```python
from build123d import *

# Parameters (mm, degrees)
BOSS_EXTRUDE3_DEPTH = 1
BOSS_EXTRUDE4_DEPTH = 3


with BuildPart() as part:
    # Sketch1 → Boss-Extrude3 (new body)
    with BuildSketch(Plane(origin=(0, 0, 0), x_dir=(1, 0, 0), z_dir=(0, 1, 0))):
        Polygon((362.222534427, 19.965180646), (284.852100337, -114.072137645), (439.598290008, -114.060221421), align=None)
        with BuildLine():
            Line((363.912669034, -12.581193275), (364.023092144, -12.093538954))
            ThreePointArc((364.023092144, -12.093538954), (365.725004108, -13.032245467), (366.663710621, -14.734157431))
            Line((366.663710621, -14.734157431), (366.1760563, -14.844580541))
            ThreePointArc((366.1760563, -14.844580541), (366.250130374, -15.507119201), (366.1760563, -16.169657861))
            Line((366.1760563, -16.169657861), (366.663710621, -16.280080971))
            ThreePointArc((366.663710621, -16.280080971), (365.725004108, -17.981992935), (364.023092144, -18.920699448))
            Line((364.023092144, -18.920699448), (363.912669034, -18.433045127))
            ThreePointArc((363.912669034, -18.433045127), (363.250130374, -18.507119201), (362.587591714, -18.433045127))
            Line((362.587591714, -18.433045127), (362.477168604, -18.920699448))
            ThreePointArc((362.477168604, -18.920699448), (360.77525664, -17.981992935), (359.836550127, -16.280080971))
            Line((359.836550127, -16.280080971), (360.324204448, -16.169657861))
            ThreePointArc((360.324204448, -16.169657861), (360.250130374, -15.507119201), (360.324204448, -14.844580541))
            Line((360.324204448, -14.844580541), (359.836550127, -14.734157431))
            ThreePointArc((359.836550127, -14.734157431), (360.77525664, -13.032245467), (362.477168604, -12.093538954))
            Line((362.477168604, -12.093538954), (362.587591714, -12.581193275))
            ThreePointArc((362.587591714, -12.581193275), (363.250130374, -12.507119201), (363.912669034, -12.581193275))
        make_face(mode=Mode.SUBTRACT)
        with BuildLine():
            ThreePointArc((313.830794955, -100.2988546), (312.128882991, -99.360148087), (311.190176478, -97.658236123))
            Line((311.190176478, -97.658236123), (311.677830799, -97.547813013))
            ThreePointArc((311.677830799, -97.547813013), (311.603756725, -96.885274353), (311.677830799, -96.222735693))
            Line((311.677830799, -96.222735693), (311.190176478, -96.112312583))
            ThreePointArc((311.190176478, -96.112312583), (312.128882991, -94.410400619), (313.830794955, -93.471694106))
            Line((313.830794955, -93.471694106), (313.941218065, -93.959348427))
            ThreePointArc((313.941218065, -93.959348427), (314.603756725, -93.885274353), (315.266295385, -93.959348427))
            Line((315.266295385, -93.959348427), (315.376718495, -93.471694106))
            ThreePointArc((315.376718495, -93.471694106), (317.078630459, -94.410400619), (318.017336972, -96.112312583))
            Line((318.017336972, -96.112312583), (317.529682651, -96.222735693))
            ThreePointArc((317.529682651, -96.222735693), (317.603756725, -96.885274353), (317.529682651, -97.547813013))
            Line((317.529682651, -97.547813013), (318.017336972, -97.658236123))
            ThreePointArc((318.017336972, -97.658236123), (317.078630459, -99.360148087), (315.376718495, -100.2988546))
            Line((315.376718495, -100.2988546), (315.266295385, -99.811200279))
            ThreePointArc((315.266295385, -99.811200279), (314.603756725, -99.885274353), (313.941218065, -99.811200279))
            Line((313.941218065, -99.811200279), (313.830794955, -100.2988546))
        make_face(mode=Mode.SUBTRACT)
        with BuildLine():
            ThreePointArc((406.858805843, -97.563455036), (407.797512356, -95.861543072), (409.49942432, -94.922836559))
            Line((409.49942432, -94.922836559), (409.60984743, -95.41049088))
            ThreePointArc((409.60984743, -95.41049088), (410.27238609, -95.336416806), (410.93492475, -95.41049088))
            Line((410.93492475, -95.41049088), (411.04534786, -94.922836559))
            ThreePointArc((411.04534786, -94.922836559), (412.747259824, -95.861543072), (413.685966337, -97.563455036))
            Line((413.685966337, -97.563455036), (413.198312016, -97.673878146))
            ThreePointArc((413.198312016, -97.673878146), (413.27238609, -98.336416806), (413.198312016, -98.998955466))
            Line((413.198312016, -98.998955466), (413.685966337, -99.109378576))
            ThreePointArc((413.685966337, -99.109378576), (412.747259824, -100.81129054), (411.04534786, -101.749997053))
            Line((411.04534786, -101.749997053), (410.93492475, -101.262342732))
            ThreePointArc((410.93492475, -101.262342732), (410.27238609, -101.336416806), (409.60984743, -101.262342732))
            Line((409.60984743, -101.262342732), (409.49942432, -101.749997053))
            ThreePointArc((409.49942432, -101.749997053), (407.797512356, -100.81129054), (406.858805843, -99.109378576))
            Line((406.858805843, -99.109378576), (407.346460164, -98.998955466))
            ThreePointArc((407.346460164, -98.998955466), (407.272389017, -98.332225876), (407.348322685, -97.665705839))
            Line((407.348322685, -97.665705839), (406.858805843, -97.563455036))
        make_face(mode=Mode.SUBTRACT)
    extrude(amount=BOSS_EXTRUDE3_DEPTH)

    # Sketch1<15> → Boss-Extrude4 (add)
    with BuildSketch(Plane(origin=(0, 0, 0), x_dir=(1, 0, 0), z_dir=(0, 1, 0))):
        with BuildLine():
            Line((315.266295385, -99.811200279), (315.376718495, -100.2988546))
            ThreePointArc((315.376718495, -100.2988546), (317.078630459, -99.360148087), (318.017336972, -97.658236123))
            Line((318.017336972, -97.658236123), (317.529682651, -97.547813013))
            ThreePointArc((317.529682651, -97.547813013), (316.725077068, -99.006594697), (315.266295385, -99.811200279))
        make_face()
        with BuildLine():
            ThreePointArc((318.017336972, -96.112312583), (317.078630459, -94.410400619), (315.376718495, -93.471694106))
            Line((315.376718495, -93.471694106), (315.266295385, -93.959348427))
            ThreePointArc((315.266295385, -93.959348427), (316.725077068, -94.76395401), (317.529682651, -96.222735693))
            Line((317.529682651, -96.222735693), (318.017336972, -96.112312583))
        make_face()
        with BuildLine():
            Line((311.677830799, -97.547813013), (311.190176478, -97.658236123))
            ThreePointArc((311.190176478, -97.658236123), (312.128882991, -99.360148087), (313.830794955, -100.2988546))
            Line((313.830794955, -100.2988546), (313.941218065, -99.811200279))
            ThreePointArc((313.941218065, -99.811200279), (312.482436381, -99.006594697), (311.677830799, -97.547813013))
        make_face()
        with BuildLine():
            ThreePointArc((313.830794955, -93.471694106), (312.128882991, -94.410400619), (311.190176478, -96.112312583))
            Line((311.190176478, -96.112312583), (311.677830799, -96.222735693))
            ThreePointArc((311.677830799, -96.222735693), (312.482436381, -94.76395401), (313.941218065, -93.959348427))
            Line((313.941218065, -93.959348427), (313.830794955, -93.471694106))
        make_face()
        with BuildLine():
            Line((407.346460164, -98.998955466), (406.858805843, -99.109378576))
            ThreePointArc((406.858805843, -99.109378576), (407.797512356, -100.81129054), (409.49942432, -101.749997053))
            Line((409.49942432, -101.749997053), (409.60984743, -101.262342732))
            ThreePointArc((409.60984743, -101.262342732), (408.151065747, -100.457737149), (407.346460164, -98.998955466))
        make_face()
        with BuildLine():
            ThreePointArc((411.04534786, -101.749997053), (412.747259824, -100.81129054), (413.685966337, -99.109378576))
            Line((413.685966337, -99.109378576), (413.198312016, -98.998955466))
            ThreePointArc((413.198312016, -98.998955466), (412.393706434, -100.457737149), (410.93492475, -101.262342732))
            Line((410.93492475, -101.262342732), (411.04534786, -101.749997053))
        make_face()
        with BuildLine():
            ThreePointArc((413.685966337, -97.563455036), (412.747259824, -95.861543072), (411.04534786, -94.922836559))
            Line((411.04534786, -94.922836559), (410.93492475, -95.41049088))
            ThreePointArc((410.93492475, -95.41049088), (412.393706434, -96.215096462), (413.198312016, -97.673878146))
            Line((413.198312016, -97.673878146), (413.685966337, -97.563455036))
        make_face()
        with BuildLine():
            Line((409.60984743, -95.41049088), (409.49942432, -94.922836559))
            ThreePointArc((409.49942432, -94.922836559), (407.797512356, -95.861543072), (406.858805843, -97.563455036))
            Line((406.858805843, -97.563455036), (407.348322685, -97.665705839))
            ThreePointArc((407.348322685, -97.665705839), (408.154031252, -96.212135097), (409.60984743, -95.41049088))
        make_face()
        with BuildLine():
            Line((360.324204448, -16.169657861), (359.836550127, -16.280080971))
            ThreePointArc((359.836550127, -16.280080971), (360.77525664, -17.981992935), (362.477168604, -18.920699448))
            Line((362.477168604, -18.920699448), (362.587591714, -18.433045127))
            ThreePointArc((362.587591714, -18.433045127), (361.128810031, -17.628439544), (360.324204448, -16.169657861))
        make_face()
        with BuildLine():
            ThreePointArc((364.023092144, -18.920699448), (365.725004108, -17.981992935), (366.663710621, -16.280080971))
            Line((366.663710621, -16.280080971), (366.1760563, -16.169657861))
            ThreePointArc((366.1760563, -16.169657861), (365.371450718, -17.628439544), (363.912669034, -18.433045127))
            Line((363.912669034, -18.433045127), (364.023092144, -18.920699448))
        make_face()
        with BuildLine():
            Line((362.587591714, -12.581193275), (362.477168604, -12.093538954))
            ThreePointArc((362.477168604, -12.093538954), (360.77525664, -13.032245467), (359.836550127, -14.734157431))
            Line((359.836550127, -14.734157431), (360.324204448, -14.844580541))
            ThreePointArc((360.324204448, -14.844580541), (361.128810031, -13.385798857), (362.587591714, -12.581193275))
        make_face()
        with BuildLine():
            ThreePointArc((366.663710621, -14.734157431), (365.725004108, -13.032245467), (364.023092144, -12.093538954))
            Line((364.023092144, -12.093538954), (363.912669034, -12.581193275))
            ThreePointArc((363.912669034, -12.581193275), (365.371450718, -13.385798857), (366.1760563, -14.844580541))
            Line((366.1760563, -14.844580541), (366.663710621, -14.734157431))
        make_face()
    extrude(amount=BOSS_EXTRUDE4_DEPTH)


solid = part.part
```
CAD build for the part. Positions are in the model's coordinates, mm. Coordinates: 2 decimals unless noted, no trailing zeros. Order: outer loops, then holes, each group sorted by start corner. A loop starts at its lowest first (then second) coordinate and runs counter-clockwise, first axis right, second up. Notation, with made-up numbers: (-6.75, 41) -> (-2.75, 41) arc R9 cw to (-2.75, 47) -> close; hole circle Ø2 at (-39, 47). An arc over 180 degrees is marked (long way). Use one line per item in the form item = value. Start each with the question number.
1) Drill centre lines: L1, parallel to X at y = 2.8, z = 96; L2, parallel to Y at x = 357, z = 7; L3, parallel to X at y = 1.9, z = 97.5. Where is each one in solid material? Low to high. Write a range as [from, to].
2) Band-saw the part on B-B on z = 5.5. Give the cut face in (x, y).
3) Band-saw the part on C-C on x = 320. Give the cut face in (y, z), then the cut area to 3 significant figures.
4) Drop a flat-ended pin along its axis: pin 1 (0.5 mm diameter, centred on x = 361, y = 0.5, fed in from +Z). Give the stop position or say it passes through.
5) Band-saw the part on A-A on y = 1.8. State how many separate pieces and enclosed holes the cut face has, then the cut area to 3 significant figures.
Entries:
q1.L1 = [311.22, 311.74], [317.47, 317.99], [407.67, 408.39], [412.15, 412.88]
q1.L2 = [0, 1]
q1.L3 = [406.87, 407.39], [413.15, 413.67]
q2.outline = (347.52, 0) -> (376.92, 0) -> (376.92, 1) -> (347.52, 1) -> close
q3.outline = (0, 53.18) -> (1, 53.18) -> (1, 114.07) -> (0, 114.07) -> close
q3.area = 60.9 mm2
q4.pin_1 = 114.07
q5.separate_pieces = 12
q5.enclosed_holes = 0
q5.area = 21.9 mm2
